Source: CAD feature listing. Evaluate the final solid. Frame: model axes, mm. A direction names the side the tool comes from. Round coordinates to 2 decimals unless told otherwise and drop trailing zeros. Write each loop counter-clockwise with the first axis right and the second up, starting at its lowest first coordinate (ties: lowest second). Pieces come first, ordered by that corner, then holes.
```python
from build123d import *

# Parameters (mm, degrees)
SKETCH1_R           = 0.5
SKETCH1_R_2         = 2.25
BOSS_EXTRUDE1_DEPTH = 1.2
SKETCH2_R           = 3.25
SKETCH2_R_2         = 1.5
BOSS_EXTRUDE2_DEPTH = 2.5
SKETCH3_R           = 2.5
CUT_EXTRUDE1_DEPTH  = 2


with BuildPart() as part:
    # Sketch1 → Boss-Extrude1 (new body)
    with BuildSketch(Plane(origin=(0, 0, 0), x_dir=(1, 0, 0), z_dir=(0, 1, 0))):
        with BuildLine():
            Line((-2.882352941, 2), (-2, 17))
            ThreePointArc((-2, 17), (0, 19), (2, 17))
            Line((2, 17), (2.882352941, 2))
            Line((2.882352941, 2), (7, 2))
            ThreePointArc((7, 2), (9, 0), (7, -2))
            Line((7, -2), (2.882352941, -2))
            Line((2.882352941, -2), (1.867646984, -14.999963756))
            ThreePointArc((1.867646984, -14.999963756), (-0.132626782, -16.99941606), (-2.132352941, -14.999416075))
            Line((-2.132352941, -14.999416075), (-2.882352941, -2))
            Line((-2.882352941, -2), (-7, -2))
            ThreePointArc((-7, -2), (-9, 0), (-7, 2))
            Line((-7, 2), (-2.882352941, 2))
        make_face()
        with Locations(Location((0, 5, 0), (0, 0, 270))):
            Circle(SKETCH1_R, mode=Mode.SUBTRACT)
        with Locations(Location((0, 7, 0), (0, 0, 270))):
            Circle(SKETCH1_R, mode=Mode.SUBTRACT)
        with Locations(Location((0, 9, 0), (0, 0, 270))):
            Circle(SKETCH1_R, mode=Mode.SUBTRACT)
        with Locations(Location((0, 11, 0), (0, 0, 270))):
            Circle(SKETCH1_R, mode=Mode.SUBTRACT)
        with Locations(Location((0, 13, 0), (0, 0, 270))):
            Circle(SKETCH1_R, mode=Mode.SUBTRACT)
        with Locations(Location((0, 15, 0), (0, 0, 270))):
            Circle(SKETCH1_R, mode=Mode.SUBTRACT)
        with Locations(Location((0, 17, 0), (0, 0, 270))):
            Circle(SKETCH1_R, mode=Mode.SUBTRACT)
        with Locations(Location((0, -15, 0), (0, 0, 90))):
            Circle(SKETCH1_R, mode=Mode.SUBTRACT)
        with Locations(Location((0, -13, 0), (0, 0, 90))):
            Circle(SKETCH1_R, mode=Mode.SUBTRACT)
        with Locations(Location((0, -11, 0), (0, 0, 90))):
            Circle(SKETCH1_R, mode=Mode.SUBTRACT)
        with Locations(Location((0, -9, 0), (0, 0, 90))):
            Circle(SKETCH1_R, mode=Mode.SUBTRACT)
        with Locations(Location((0, -7, 0), (0, 0, 90))):
            Circle(SKETCH1_R, mode=Mode.SUBTRACT)
        with Locations(Location((0, -5, 0), (0, 0, 90))):
            Circle(SKETCH1_R, mode=Mode.SUBTRACT)
        with Locations(Location((7, 0, 0), (0, 0, 270))):
            Circle(SKETCH1_R, mode=Mode.SUBTRACT)
        with Locations(Location((5, 0, 0), (0, 0, 270))):
            Circle(SKETCH1_R, mode=Mode.SUBTRACT)
        with Locations(Location((-5, 0, 0), (0, 0, 90))):
            Circle(SKETCH1_R, mode=Mode.SUBTRACT)
        with Locations(Location((-7, 0, 0), (0, 0, 90))):
            Circle(SKETCH1_R, mode=Mode.SUBTRACT)
        with Locations(Location((0, 0, 0), (0, 0, 270))):
            Circle(SKETCH1_R_2, mode=Mode.SUBTRACT)
    extrude(amount=BOSS_EXTRUDE1_DEPTH)

    # Sketch2 → Boss-Extrude2 (add)
    with BuildSketch(Plane(origin=(0, 0, 0), x_dir=(1, 0, 0), z_dir=(0, 1, 0))):
        with Locations(Location((0, 0, 0), (0, 0, 270))):
            Circle(SKETCH2_R)
        with Locations(Location((0, 0, 0), (0, 0, 270))):
            Circle(SKETCH2_R_2, mode=Mode.SUBTRACT)
    extrude(amount=-BOSS_EXTRUDE2_DEPTH)

    # Sketch3 → Cut-Extrude1 (cut)
    with BuildSketch(Plane.XZ.offset(2.5)):
        with Locations(Location((0, 0, 0), (0, 0, 270))):
            Circle(SKETCH3_R)
    extrude(amount=-CUT_EXTRUDE1_DEPTH, mode=Mode.SUBTRACT)


solid = part.part
```
Q1. Pin query (flat end, axial travel): P1, Ø9, axis at x = 2.5, z = -4, coming from the -Y side; P2, Ø4, axis at x = 0, z = 0, coming from the +Y side; P3, Ø0.6, axis at x = 5.5, y = 0.5, coming from the +Z side; P4, Ø1.3, axis at x = -5, y = 1, coming from the -Z side. Return the tip coordinate at first contact, or that it passes through.
Q2. Set-up query: faces 4 (the face through (5, 1, 2)), 5 (the face through (-2.44, -1.51, 0.54)), 6 (the face through (-5, 1, -2)), 7 (the face through (-5, 1, 2)), 8 (the face through (0.676, 0.592, 2.146)). Return all of +Z, -Z, +X, -X, +Y, -Y with unobstructed straight access to the full face (end or side cutting, diameter ignored); none if empty.
Q3. Section query C-C, the plane z = 0. Give the number of separate pieces and of enclosed holes in the cut face, and give its area (4 significant figures).
Q4. Section query A-A, the plane x = -5. Output: boundary loops of the cut face in (y, z), and give its area (3 significant figures).
Q5. Mould query, pull axis X, two halves, no side actions, for faces 1 (the face through (9, 1, 0)), 2 (the face through (0, 0, -4)), 3 (the face through (0, 0.6, -9.5)). Classes: pulls with the +X half, pulls with the -X half, needs draft (parallel to the pull), parting line crosses it, or undercut.
Q6. Section query B-B, the plane z = 11. Output: boundary loops of the cut face in (x, y).
Q7. Line query: line 1 (X direction, y = 0.95, z = 0); line 2 (Z direction, x = -5, y = 0.6); line 3 (X direction, y = -2.05, z = -1.5). Output: solid intervals per line, ascending.
Filled in:
1. P1: stops at y = -2.5
1. P2: stops at y = 0
1. P3: stops at z = 2
1. P4: stops at z = -2
2. face 4: +Z, +X, +Y, -Y
2. face 5: -Y
2. face 6: -Z, -X, +Y, -Y
2. face 7: +Z, -X, +Y, -Y
2. face 8: +Y
3. separate pieces: 6
3. enclosed holes: 0
3. area: 16.15 mm2
4. outline: (0, -2) - (1.2, -2) - (1.2, -0.5) - (0, -0.5) - close; (0, 0.5) - (1.2, 0.5) - (1.2, 2) - (0, 2) - close
4. area: 3.60 mm2
5. face 1: pulls with the +X half
5. face 2: needs draft
5. face 3: undercut
6. outline: (-2.36, 0) - (-0.5, 0) - (-0.5, 1.2) - (-2.36, 1.2) - close; (0.5, 0) - (2.18, 0) - (2.18, 1.2) - (0.5, 1.2) - close
7. line 1: x = -9 to -7.5, -6.5 to -5.5, -4.5 to -2.25, 2.25 to 4.5, 5.5 to 6.5, 7.5 to 9
7. line 2: z = -2 to -0.5, 0.5 to 2
7. line 3: x = -2.88 to -2, 2 to 2.88
